Could you check a few things on this model? Use its own coordinates, in mm. A direction names the side the tool comes from. Coordinates: 2 decimals unless noted, no trailing zeros. Loops run counter-clockwise (first coordinate to the right, second up) from the corner with the lowest first, then second, coordinate; pieces in that order, holes last. Notation, with made-up numbers: M 37,65.25 L 64,65.25 A30 ccw 64,88.25 Z; hole C -16,-34.75 d1. An arc over 180 degrees is marked long. Write each question's results on one line, items separated by ' | '.
```python
from build123d import *

# Parameters (mm, degrees)
BOSS_EXTRUDE2_DEPTH  = 6.35
CUT_EXTRUDE1_START   = -12.7
CUT_EXTRUDE1_DEPTH   = 12.7
SKETCH17_W           = 6.35
SKETCH17_H           = 9.525
CUT_EXTRUDE2_DEPTH   = 2.8575
M2_CLEARANCE_HOLE1_D = 2.6
M3_CLEARANCE_HOLE1_D = 3.2


with BuildPart() as part:
    # Sketch5 → Boss-Extrude2 (new body)
    with BuildSketch(Plane(origin=(0, 0, 0), x_dir=(0, 0, -1), z_dir=(1, 0, 0))):
        Polygon((-11.43, 5.08), (-2.54, 5.08), (-6.35, 0), (-6.35, -9.525), (6.35, -9.525), (6.35, 0), (2.54, 5.08), (11.43, 5.08), (13.335, 10.16), (13.335, 33.02), (6.985, 33.02), (6.985, 10.16), (-6.985, 10.16), (-6.985, 33.02), (-13.335, 33.02), (-13.335, 10.16), align=None)
    extrude(amount=BOSS_EXTRUDE2_DEPTH)

    # Cut-Extrude1: read off the stored shape, not the designer's step
    # Cut-Extrude1 outline → Cut-Extrude1 (cut)
    with BuildSketch(Plane.XY.offset(6.35).offset(CUT_EXTRUDE1_START)):
        with BuildLine():
            Line((6.35, -9.525), (6.35, -6.35))
            ThreePointArc((6.35, -6.35), (5.42006403, -8.59506403), (3.175, -9.525))
            Line((3.175, -9.525), (6.35, -9.525))
        make_face()
        with BuildLine():
            Line((0, -9.525), (3.175, -9.525))
            ThreePointArc((3.175, -9.525), (0.92993597, -8.59506403), (0, -6.35))
            Line((0, -6.35), (0, -9.525))
        make_face()
    extrude(amount=CUT_EXTRUDE1_DEPTH, mode=Mode.SUBTRACT)

    # Sketch17 → Cut-Extrude2 (cut, symmetric)
    with BuildSketch(Plane.XY):
        with Locations((3.175, -4.7625)):
            Rectangle(SKETCH17_W, SKETCH17_H)
    extrude(amount=CUT_EXTRUDE2_DEPTH, both=True, mode=Mode.SUBTRACT)

    # M2 Clearance Hole1 (through all)
    with Locations(Plane(origin=(6.35, 0, 0), x_dir=(0, 0, -1), z_dir=(1, 0, 0))):
        with Locations((-10.159977629, 17.689823395), (-10.159977629, 30.389823395), (10.160022371, 30.389823395), (10.160022371, 17.689823395)):
            Hole(M2_CLEARANCE_HOLE1_D / 2)

    # M3 Clearance Hole1 (through all)
    with Locations(Plane.XY.offset(6.35)):
        with Locations((3.175, -6.35)):
            Hole(M3_CLEARANCE_HOLE1_D / 2)


solid = part.part
```
(1) Please list where these lines run through material, in increasing order: probe 1 along Z at (x, y) = (4.5, 20.5) (3 decimals); probe 2 along Z at (x, y) = (2, 16.5) (3 decimals); probe 3 along Z at (x, y) = (3, -2). Write a range as from..to.
Reported:
probe 1: z = -13.335..-6.985, 6.985..13.335 | probe 2: z = -13.335..-10.684, -9.636..-6.985, 6.985..9.636, 10.684..13.335 | probe 3: z = -6.35..-2.86, 2.86..6.35
(2) Imagine slicing it at C-C, the plane z = 10.5. List the corners of the cut face in (x, y) for me, and give its area (3 significant figures).
Reported:
outline: M 0,5.08 L 6.35,5.08 L 6.35,16.44 L 0,16.44 Z; M 0,18.94 L 6.35,18.94 L 6.35,29.14 L 0,29.14 Z; M 0,31.64 L 6.35,31.64 L 6.35,33.02 L 0,33.02 Z | area: 146 mm2
(3) Imagine slicing it at A-A, the plane z = 5.5. List the corners of the cut face in (x, y) for me (3 decimals), and give its area (3 significant figures).
Reported:
outline: M 0,-6.35 A3.175 ccw 6.35,-6.35 L 6.35,1.133 L 0,1.133 Z; M 0,5.08 L 6.35,5.08 L 6.35,10.16 L 0,10.16 Z; hole C 3.175,-6.35 d3.2 | area: 87.6 mm2
(4) Which directions (+Z, -Z, +X, -X, +Y, -Y) give clear straight access to the entire face, cutting with the end or side of a thin tool? Please do faces 5 (the flat face through (3, -4, 2.858)), 6 (the flat face through (3, 10.16, 0)), 7 (the flat face through (3, 5.08, 7)), 8 (the flat face through (3, 5.08, -7)), 9 (the cylindrical face through (3.13, 29.12, 9.88)).
Reported:
face 5: +X, -X, -Y | face 6: +X, -X, +Y | face 7: +Z, +X, -X | face 8: -Z, +X, -X | face 9: +X, -X
(5) Will these pins go through, and if not, where does the flat tip stop? P1, Ø1, axis at x = 4, z = -6, coming from the -Y side; P2, Ø3, axis at x = 4, y = -3, coming from the +Z side; P3, Ø1.7, axis at x = 3.5, z = -1, coming from the -Y side.
Reported:
P1: stops at y = -9.51 | P2: stops at z = 6.35 | P3: stops at y = 0
(6) If we mould it in two halves opening along X, with no side actions, what happens to faces 1 (the flat face through (6.35, 9, 0)), 2 (the cylindrical face through (4.354, -5.269, -4.628)), 3 (the flat face through (0, 9, 0)), 4 (the flat face through (3.1, 2.6, 4.4))? For each: released by +X, released by -X, zero draft, split by the parting line, or undercut.
Reported:
face 1: released by +X | face 2: undercut | face 3: released by -X | face 4: zero draft
(7) Imagine slicing it at B-B, the plane y = 17. List the corners of the cut face in (x, z) for me (3 decimals), and give its area (3 significant figures).
Reported:
outline: M 0,-13.335 L 6.35,-13.335 L 6.35,-11.262 L 0,-11.262 Z; M 0,-9.058 L 6.35,-9.058 L 6.35,-6.985 L 0,-6.985 Z; M 0,6.985 L 6.35,6.985 L 6.35,9.058 L 0,9.058 Z; M 0,11.262 L 6.35,11.262 L 6.35,13.335 L 0,13.335 Z | area: 52.7 mm2
(8) Imagine slicing it at D-D, the plane z = -5.25. List the corners of the cut face in (x, y) for me (3 decimals).
Reported:
outline: M 0,-6.35 A3.175 ccw 6.35,-6.35 L 6.35,1.467 L 0,1.467 Z; M 0,5.08 L 6.35,5.08 L 6.35,10.16 L 0,10.16 Z; hole C 3.175,-6.35 d3.2
